Model file for the job. Use its own axes, mm. A direction names the side the tool comes from. Give positions to 0.01 mm unless a question says otherwise; leave off trailing zeros. Loops run counter-clockwise (first coordinate to the right, second up) from the corner with the lowest first, then second, coordinate; pieces in that order, holes last. Notation, with made-up numbers: M 19,-8.5 L 76,-8.5 A33 ccw 76,28.5 Z; hole C 78,27 d7. An arc over 180 degrees is marked long. Answer in a Markdown table with one row per item.
```python
from build123d import *

# Parameters (mm, degrees)
RESSALTO_EXTRUS_O1_DEPTH = 1.5
CORTE_EXTRUS_O1_REACH    = 3.5
ESBO_O2_R                = 2.1
CORTE_EXTRUS_O2_DEPTH    = 10


with BuildPart() as part:
    # Esboço1 → Ressalto-extrusão1 (new body)
    with BuildSketch(Plane.XY):
        Polygon((56.463679973, 135.159747673), (-55.864365487, 135.159747673), (-94.700342757, 88.87683224), (-94.700342757, 23.490318666), (-49.700342757, -30.138593001), (-49.700342757, -133.732537696), (-48.380219867, -134.840252327), (48.979534352, -134.840252327), (50.299657243, -133.732537696), (50.299657243, -30.138593001), (95.299657243, 23.490318666), (95.299657243, 88.87683224), align=None)
    extrude(amount=RESSALTO_EXTRUS_O1_DEPTH)

    # Esboço2 → Corte-extrusão1 (cut, up to next)
    with BuildSketch(Plane.XY.offset(1.5), mode=Mode.PRIVATE) as corte_extrus_o1_sk1:
        with Locations((-71.672714117, 109.298736063)):
            Circle(ESBO_O2_R)
    corte_extrus_o1_tool1 = extrude(corte_extrus_o1_sk1.sketch, amount=-CORTE_EXTRUS_O1_REACH, mode=Mode.PRIVATE) & part.part
    add(corte_extrus_o1_tool1.solids().sort_by_distance((-71.672714, 109.298736, 1.5))[0], mode=Mode.SUBTRACT)
    # Esboço2 → Corte-extrusão1 (cut, up to next)
    with BuildSketch(Plane.XY.offset(1.5), mode=Mode.PRIVATE) as corte_extrus_o1_sk2:
        with Locations((-45.200342757, -129.610252327)):
            Circle(ESBO_O2_R)
    corte_extrus_o1_tool2 = extrude(corte_extrus_o1_sk2.sketch, amount=-CORTE_EXTRUS_O1_REACH, mode=Mode.PRIVATE) & part.part
    add(corte_extrus_o1_tool2.solids().sort_by_distance((-45.200343, -129.610252, 1.5))[0], mode=Mode.SUBTRACT)
    # Esboço2 → Corte-extrusão1 (cut, up to next)
    with BuildSketch(Plane.XY.offset(1.5), mode=Mode.PRIVATE) as corte_extrus_o1_sk3:
        with Locations((45.799657243, -129.610252327)):
            Circle(ESBO_O2_R)
    corte_extrus_o1_tool3 = extrude(corte_extrus_o1_sk3.sketch, amount=-CORTE_EXTRUS_O1_REACH, mode=Mode.PRIVATE) & part.part
    add(corte_extrus_o1_tool3.solids().sort_by_distance((45.799657, -129.610252, 1.5))[0], mode=Mode.SUBTRACT)
    # Esboço2 → Corte-extrusão1 (cut, up to next)
    with BuildSketch(Plane.XY.offset(1.5), mode=Mode.PRIVATE) as corte_extrus_o1_sk4:
        with Locations((72.272028603, 109.298736063)):
            Circle(ESBO_O2_R)
    corte_extrus_o1_tool4 = extrude(corte_extrus_o1_sk4.sketch, amount=-CORTE_EXTRUS_O1_REACH, mode=Mode.PRIVATE) & part.part
    add(corte_extrus_o1_tool4.solids().sort_by_distance((72.272029, 109.298736, 1.5))[0], mode=Mode.SUBTRACT)
    # Esboço2 → Corte-extrusão1 (cut, up to next)
    with BuildSketch(Plane.XY.offset(1.5), mode=Mode.PRIVATE) as corte_extrus_o1_sk5:
        with Locations((-68.753142763, -0.431592924)):
            Circle(ESBO_O2_R)
    corte_extrus_o1_tool5 = extrude(corte_extrus_o1_sk5.sketch, amount=-CORTE_EXTRUS_O1_REACH, mode=Mode.PRIVATE) & part.part
    add(corte_extrus_o1_tool5.solids().sort_by_distance((-68.753143, -0.431593, 1.5))[0], mode=Mode.SUBTRACT)
    # Esboço2 → Corte-extrusão1 (cut, up to next)
    with BuildSketch(Plane.XY.offset(1.5), mode=Mode.PRIVATE) as corte_extrus_o1_sk6:
        with Locations((69.352457249, -0.431592924)):
            Circle(ESBO_O2_R)
    corte_extrus_o1_tool6 = extrude(corte_extrus_o1_sk6.sketch, amount=-CORTE_EXTRUS_O1_REACH, mode=Mode.PRIVATE) & part.part
    add(corte_extrus_o1_tool6.solids().sort_by_distance((69.352457, -0.431593, 1.5))[0], mode=Mode.SUBTRACT)

    # Esboço3 → Corte-extrusão2 (cut)
    with BuildSketch(Plane.XY.offset(1.5)):
        Polygon((-53.532827197, 130.159747673), (-64.879577854, 116.637216813), (-64.263293687, 109.593056549), (-70.675930858, 101.950773162), (-77.720091122, 101.334488995), (-89.700342757, 87.056981069), (-89.700342757, 25.310169837), (-74.789956765, 7.540663764), (-67.745796501, 6.924379597), (-61.334000151, -0.716901738), (-61.950284318, -7.761062002), (-44.700342757, -28.318741829), (-44.700342757, -117.173246706), (-31.407709232, -128.327090595), (32.007023717, -128.327090595), (45.299657243, -117.173246706), (45.299657243, -28.318741829), (62.549598803, -7.761062002), (61.933314636, -0.716901738), (68.345110987, 6.924379597), (75.389271251, 7.540663764), (90.299657243, 25.310169837), (90.299657243, 87.056981069), (78.319405608, 101.334488995), (71.275245343, 101.950773162), (64.862608173, 109.593056549), (65.47889234, 116.637216813), (54.132141682, 130.159747673), align=None)
    extrude(amount=-CORTE_EXTRUS_O2_DEPTH, mode=Mode.SUBTRACT)


solid = part.part
```
(1) Flat gauge pins, fed straight in: P1, Ø5.5, axis at x = 72.27, y = 109.3, coming from the -Z side; P2, Ø0.8, axis at y = -90.5, z = 1, coming from the +X side; P3, Ø2.5, axis at x = 45.8, y = -129.61, coming from the -Z side. Where does each tip first touch, or does it go through?
Established:
| item | result |
|---|---|
| P1 | stops at z = 0 |
| P2 | stops at x = 50.3 |
| P3 | passes through |
(2) Which spindle directions (+Z, -Z, +X, -X, +Y, -Y) get a long thin tool onto all of the face, cutting with end or side? Do faces 1 (the flat face through (-49, -29, 0)), 2 (the flat face through (53.804, -18.184, 0.76)). Say none if no direction does.
Established:
| item | result |
|---|---|
| face 1 | -Z, +X, -X, +Y, -Y |
| face 2 | +Z, -Z |
(3) Mould opens along X. For faces 3 (the flat face through (-72.515, -2.949, 0.74)), 4 (the flat face through (72.485, -3.7, 0.74)), 5 (the flat face through (-49, -29, 1.5)), 6 (the flat face through (84.39, 94.1, 0.76)) say: pulls with the +X half, pulls with the -X half, needs draft (parallel to the pull), parting line crosses it, or undercut.
Established:
| item | result |
|---|---|
| face 3 | pulls with the -X half |
| face 4 | pulls with the +X half |
| face 5 | needs draft |
| face 6 | undercut |
(4) Saw through at C-C, the plane z = 0.4. Count the separate pieces of the cut face and the enclosed holes in it, and give its area (3 significant figures).
Established:
| item | result |
|---|---|
| separate pieces | 1 |
| enclosed holes | 7 |
| area | 4,470 mm2 |
(5) Saw through at B-B, the plane x = 39. Give the cut face in (y, z), and give its area (3 significant figures).
Established:
| item | result |
|---|---|
| outline | M -134.84,0 L -122.46,0 L -122.46,1.5 L -134.84,1.5 Z; M 130.16,0 L 135.16,0 L 135.16,1.5 L 130.16,1.5 Z |
| area | 26.1 mm2 |
(6) Saw through at A-A, the plane y = -108. Give the cut face in (x, z).
Established:
| item | result |
|---|---|
| outline | M -49.7,0 L -44.7,0 L -44.7,1.5 L -49.7,1.5 Z; M 45.3,0 L 50.3,0 L 50.3,1.5 L 45.3,1.5 Z |
(7) Wall check: L1, parallel to X at y = -74.5, z = 0.1; L2, parallel to X at y = 35, z = 1.2; L3, parallel to Y at x = 12, z = 1.05. Give the ranges that are in metal, low to high.
Established:
| item | result |
|---|---|
| L1 | x = -49.7 to -44.7, 45.3 to 50.3 |
| L2 | x = -94.7 to -89.7, 90.3 to 95.3 |
| L3 | y = -134.84 to -128.33, 130.16 to 135.16 |
